Could you check a few things on this model? Use its own coordinates, in mm. Round coordinates to 2 decimals unless told otherwise and drop trailing zeros. Loops run counter-clockwise (first coordinate to the right, second up) from the corner with the lowest first, then second, coordinate; pieces in that order, holes last. Notation, with made-up numbers: M 69,37.25 L 88,37.25 A19 ccw 88,43.25 Z; hole C 89,6.5 d4. An arc over 180 degrees is marked long. One line per item, written item: value. Start each with the question number.
Q1. Please list where these lines run through material, in increasing order: line 1 along Z through (x, y) = (-19, 14.25); line 2 along Y through (x, z) = (-22, 34); line 3 along Z through (x, y) = (-32, 18.25).
Q2. Imagine slicing it at D-D (y = 22.5). Please give me the cut outline in (x, z).
Q3. Thinking about a two-plate mould opening in Y: for faces 1 (the face through (-42, 0, 3)), 2 (the face through (-31.79, 13.07, 36.17)), 3 (the face through (-32, 13, 39.471)), which applies, released by +Y, released by -Y, zero draft, split by the parting line, or undercut?
Q4. Imagine slicing it at B-B (x = -25). Please give me the cut outline in (y, z).
Q5. Imagine slicing it at C-C (x = -34). Please give me the cut outline in (y, z).
Q6. Imagine slicing it at A-A (y = 13). Please give me the cut outline in (x, z).
Q7. I'm going to push a flat-ended pin straight in: pin 1 Ø10 at (y, z) = (22.5, 16.5) entering from +X. Where does the tip first touch, or does it pass through?
from build123d import *

# Parameters (mm, degrees)
BOSS_EXTRUDE1_DEPTH = 26
SKETCH2_R           = 1.7
CUT_EXTRUDE1_DEPTH  = 31
CUT_EXTRUDE2_DEPTH  = 1


with BuildPart() as part:
    # Sketch1 → Boss-Extrude1 (new body)
    with BuildSketch(Plane(origin=(0, 0, 0), x_dir=(1, 0, 0), z_dir=(0, 1, 0))):
        with BuildLine():
            Line((-46.998275301, 32.528571429), (-46.998275301, -39.471428571))
            Line((-46.998275301, -39.471428571), (-16.998275301, -39.471428571))
            Line((-16.998275301, -39.471428571), (-16.998275301, -26.471428571))
            ThreePointArc((-16.998275301, -26.471428571), (-39.998275301, -3.471428571), (-16.998275301, 19.528571429))
            Line((-16.998275301, 19.528571429), (-16.998275301, 32.528571429))
            Line((-16.998275301, 32.528571429), (-46.998275301, 32.528571429))
        make_face()
    extrude(amount=BOSS_EXTRUDE1_DEPTH)

    # Sketch2 → Cut-Extrude1 (cut, through all)
    with BuildSketch(Plane(origin=(-16.998275301, 0, 0), x_dir=(0, 0, -1), z_dir=(1, 0, 0))):
        with Locations((-34.471428571, 13)):
            Circle(SKETCH2_R)
        with Locations((27.528571429, 13)):
            Circle(SKETCH2_R)
    extrude(amount=-CUT_EXTRUDE1_DEPTH, mode=Mode.SUBTRACT)

    # Sketch3 → Cut-Extrude2 (cut)
    with BuildSketch(Plane(origin=(-16.998275301, 0, 0), x_dir=(0, 0, -1), z_dir=(1, 0, 0))):
        Polygon((-34.164231178, 21.664809495), (-32.617436306, 21.664809495), (-32.617436306, 21.33916847), (-33.87929528, 21.33916847), (-33.87929528, 20.362245393), (-32.617436306, 20.362245393), (-32.617436306, 20.036604367), (-33.87929528, 20.036604367), (-33.87929528, 18.489809495), (-34.164231178, 18.489809495), align=None)
        with BuildLine():
            Line((-31.925449127, 20.687886418), (-32.210385024, 20.687886418))
            add(Edge.make_bspline(
                [(-32.210385024, 20.687886418), (-32.208527964, 20.725687867), (-32.204880747, 20.799928905), (-32.187800799, 20.908172734), (-32.163361574, 21.01163673), (-32.128807184, 21.109490152), (-32.085893632, 21.202598213), (-32.034431393, 21.290591084), (-31.973476971, 21.373133091), (-31.904346577, 21.449459042), (-31.829263597, 21.519479196), (-31.748250352, 21.579945023), (-31.663119506, 21.631033196), (-31.574129337, 21.673742608), (-31.480275826, 21.705800897), (-31.382410662, 21.72958767), (-31.280103874, 21.74389907), (-31.210398997, 21.745437389), (-31.174948325, 21.746219752)],
                knots=[0, 0, 0, 0, 0.000113468, 0.000222848, 0.000328209, 0.000432002, 0.000533594, 0.000635367, 0.000737261, 0.00084084, 0.000943908, 0.001044781, 0.001143495, 0.001241361, 0.001340322, 0.001440438, 0.001543158, 0.001649467, 0.001649467, 0.001649467, 0.001649467], degree=3))
            add(Edge.make_bspline(
                [(-31.174948325, 21.746219752), (-31.140133929, 21.745404723), (-31.071724885, 21.743803222), (-30.971882915, 21.730050002), (-30.876834941, 21.708509359), (-30.786766753, 21.678287517), (-30.702396966, 21.637661643), (-30.623091775, 21.58885959), (-30.54790704, 21.532417315), (-30.480228029, 21.465965641), (-30.418081414, 21.395024907), (-30.364467225, 21.319289451), (-30.318553856, 21.241067171), (-30.280283603, 21.159761588), (-30.252111249, 21.074607155), (-30.230722446, 20.986843621), (-30.218632577, 20.895562542), (-30.216777086, 20.833780167), (-30.215833742, 20.802369592)],
                knots=[0, 0, 0, 0, 0.000104402, 0.000205146, 0.000301729, 0.000396461, 0.000489487, 0.000581988, 0.000675485, 0.000770845, 0.000865978, 0.000958102, 0.001048749, 0.001137814, 0.001227115, 0.00131736, 0.00140848, 0.001502716, 0.001502716, 0.001502716, 0.001502716], degree=3))
            add(Edge.make_bspline(
                [(-30.215833742, 20.802369592), (-30.21736377, 20.75814655), (-30.220396976, 20.67047652), (-30.24657322, 20.541476852), (-30.287015551, 20.416377263), (-30.336067513, 20.315703408), (-30.385616171, 20.234988656), (-30.429322129, 20.16793661), (-30.481621049, 20.096429789), (-30.542034416, 20.019747997), (-30.609650855, 19.937656676), (-30.684957018, 19.850122138), (-30.76852818, 19.758074075), (-30.827182388, 19.695203802), (-30.857575529, 19.662626002)],
                knots=[0, 0, 0, 0, 0.00013255, 0.000262774, 0.000393306, 0.000526148, 0.000597485, 0.000677395, 0.000766194, 0.000863145, 0.000970232, 0.001085232, 0.001209518, 0.00134318, 0.00134318, 0.00134318, 0.00134318], degree=3))
            Line((-30.857575529, 19.662626002), (-31.651961546, 18.815450521))
            Line((-31.651961546, 18.815450521), (-30.175128614, 18.815450521))
            Line((-30.175128614, 18.815450521), (-30.175128614, 18.489809495))
            Line((-30.175128614, 18.489809495), (-32.332500409, 18.489809495))
            Line((-32.332500409, 18.489809495), (-31.10117028, 19.803821915))
            add(Edge.make_bspline(
                [(-31.10117028, 19.803821915), (-31.071191126, 19.835116808), (-31.013607306, 19.895227891), (-30.932161682, 19.982987576), (-30.8590106, 20.064403231), (-30.793680537, 20.139321029), (-30.737588714, 20.208836808), (-30.687811761, 20.270699146), (-30.647928689, 20.327626398), (-30.604644008, 20.393612526), (-30.562721325, 20.474177985), (-30.526696545, 20.572633546), (-30.504730218, 20.673986125), (-30.502095118, 20.742477259), (-30.500769639, 20.776928886)],
                knots=[0, 0, 0, 0, 0.000130011, 0.000249724, 0.000359165, 0.000458368, 0.000547868, 0.000627136, 0.000696488, 0.000756294, 0.000863824, 0.000968046, 0.001070082, 0.001173354, 0.001173354, 0.001173354, 0.001173354], degree=3))
            add(Edge.make_bspline(
                [(-30.500769639, 20.776928886), (-30.501346348, 20.798592726), (-30.502482931, 20.841287995), (-30.512513843, 20.903886076), (-30.527672659, 20.964269872), (-30.549394429, 21.022625119), (-30.578066257, 21.078365103), (-30.612967109, 21.131557675), (-30.653235238, 21.182982665), (-30.699818175, 21.231200299), (-30.750991482, 21.275361107), (-30.80505198, 21.314480813), (-30.862247432, 21.347173435), (-30.922336686, 21.373973608), (-30.985152219, 21.394996989), (-31.050815523, 21.409564415), (-31.119145166, 21.418710668), (-31.165802695, 21.419948167), (-31.189576731, 21.420578726)],
                knots=[0, 0, 0, 0, 6.4952e-05, 0.000128007, 0.000189711, 0.000251496, 0.000314359, 0.000377338, 0.000442102, 0.000510025, 0.000578115, 0.000644657, 0.000709898, 0.00077538, 0.000841751, 0.000908254, 0.000976888, 0.001048193, 0.001048193, 0.001048193, 0.001048193], degree=3))
            add(Edge.make_bspline(
                [(-31.189576731, 21.420578726), (-31.214405986, 21.41993009), (-31.263166544, 21.418656275), (-31.334757381, 21.409745715), (-31.403052336, 21.394373417), (-31.468223206, 21.373348863), (-31.530380258, 21.346625751), (-31.589221213, 21.313341097), (-31.644613976, 21.273623213), (-31.69666268, 21.228592137), (-31.744617861, 21.178456528), (-31.786751812, 21.12256749), (-31.823567311, 21.061945477), (-31.855688544, 20.996754063), (-31.881774063, 20.926401706), (-31.90170685, 20.851138145), (-31.917479203, 20.771290178), (-31.922748361, 20.716149422), (-31.925449127, 20.687886418)],
                knots=[0, 0, 0, 0, 7.4482e-05, 0.00014627, 0.000216015, 0.0002842, 0.000351428, 0.000418642, 0.000486589, 0.000555575, 0.000624857, 0.000694312, 0.000765104, 0.000837353, 0.000912017, 0.000989777, 0.001070732, 0.001155858, 0.001155858, 0.001155858, 0.001155858], degree=3))
        make_face()
    extrude(amount=-CUT_EXTRUDE2_DEPTH, mode=Mode.SUBTRACT)


solid = part.part
Report:
1. line 1: z = -32.53 to -28.68, -26.38 to -19.44, 26.38 to 33.32, 35.62 to 39.47
1. line 2: y = 0 to 11.37, 14.63 to 26
1. line 3: z = -32.53 to -13.96, 20.91 to 39.47
2. outline: M -47,-32.53 L -17,-32.53 L -17,-19.53 A23 cw -17,26.47 L -17,39.47 L -47,39.47 Z
3. face 1: released by -Y
3. face 2: undercut
3. face 3: zero draft
4. outline: M 0,-32.53 L 26,-32.53 L 26,-18.09 L 0,-18.09 Z; M 0,25.03 L 26,25.03 L 26,39.47 L 0,39.47 Z; hole C 13,-27.53 d3.4; hole C 13,34.47 d3.4
5. outline: M 0,-32.53 L 26,-32.53 L 26,-12.02 L 0,-12.02 Z; M 0,18.96 L 26,18.96 L 26,39.47 L 0,39.47 Z; hole C 13,-27.53 d3.4; hole C 13,34.47 d3.4
6. outline: M -47,-32.53 L -17,-32.53 L -17,-29.23 L -47,-29.23 Z; M -47,-25.83 L -17,-25.83 L -17,-19.53 A23 cw -17,26.47 L -17,32.77 L -47,32.77 Z; M -47,36.17 L -17,36.17 L -17,39.47 L -47,39.47 Z
7. pin 1: stops at x = -31.28
